Autodesk Inventor part; units mm, degrees
ref_plane "YZ Plane" through (0, 0, 0) normal (1, 0, 0) x (0, 1, 0)
ref_plane "XZ Plane" through (0, 0, 0) normal (0, 1, 0) x (-1, 0, 0)
ref_plane "XY Plane" through (0, 0, 0) normal (0, 0, 1) x (1, 0, 0)
sketch "Skizze1" plane through (0, 0, 0) normal (0, 0, 1) x (1, 0, 0)
  circle A0 centre (0, 0) radius 7.6
  line L0 (-22.5, 20) -> (-22.5, -20)
  line L1 (-22.5, -20) -> (-17.5, -20)
  line L2 (-17.5, -20) -> (-17.5, -10)
  line L3 (-22.5, 20) -> (-17.5, 20)
  line L4 (-17.5, 20) -> (-17.5, 10)
  line L5 (-17.5, 10) -> (0, 10)
  line L6 (-17.5, -10) -> (0, -10)
  arc A1 (0, -10) -> (0, 10) centre (0, 0) ccw
  dimension "d0" = 15.2
  dimension "d23" = 5
  dimension "d24" = 10
  dimension "d25" = 5
  dimension "d26" = 10
  dimension "d27" = 40
  dimension "d28" = 20
  dimension "d38" = 22.5
extrude "Extrusion1" add sketch "Skizze1" along normal blind 24
sketch "Skizze2" plane through (-22.5, -20, 0) normal (-1, 0, 0) x (0, 0, 1)
  line L0 (0, 40) -> (0, 0)
  line L1 (0, 0) -> (24, 0)
  line L2 (0, 40) -> (5, 40)
  line L3 (5, 40) -> (5, 0)
  line L4 (5, 0) -> (0, 0)
  line L5 (0, 0) -> (0, 40)
  point P0 (0, 20)
  dimension "d12" = 5
extrude "Extrusion2" add sketch "Skizze2" along normal blind 20
sketch "Skizze3" plane through (-22.5, -20, 5) normal (0, 0, 1) x (1, 0, 0)
  circle A0 centre (-10, 30) radius 1.6
  line L0 (0, 40) -> (-20, 40)
  line L1 (-20, 0) -> (-20, 40)
  circle A1 centre (-10, 10) radius 1.6
  line L2 (0, 0) -> (-20, 0)
  point P0 (22.5, 20)
  dimension "d15" = 3.2
  dimension "d16" = 10
  dimension "d17" = 10
  dimension "d18" = 3.2
  dimension "d19" = 10
  dimension "d20" = 10
extrude "Extrusion3" cut sketch "Skizze3" against normal through all
fillet "Rundung1" radius 2 6 edges at (-17.5, -10, 12) (-17.5, 10, 12) (-17.5, 20, 12) (-17.5, -20, 12) (-42.5, -20, 2.5) (-42.5, 20, 2.5)
sketch "Skizze4" plane through (-17.5, -18, 0) normal (1, 0, 0) x (0, 0, -1)
  circle A0 centre (-15, 3) radius 1.6
  circle A1 centre (-15, 33) radius 1.6
  line L0 (0, 0) -> (0, 6)
  line L1 (-24, -2) -> (0, -2)
  line L2 (-5, 38) -> (-24, 38)
  point P0 (0, 18)
  dimension "d30" = 3.2
  dimension "d31" = 3.2
  dimension "d32" = 15
  dimension "d33" = 5
  dimension "d34" = 15
  dimension "d35" = 5
extrude "Extrusion4" cut sketch "Skizze4" against normal through all
sketch "Skizze5" plane through (0, 0, 24) normal (0, 0, 1) x (1, 0, 0)
  circle A0 centre (0, 0) radius 7.6
  circle A1 centre (0, 0) radius 10
extrude "Extrusion5" add sketch "Skizze5" along normal blind 21
properties part number "flange" material "ABS-Kunststoff"
Source: CAD feature listing. Evaluate the final solid. Frame: model axes, mm. A direction names the side the tool comes from. Round coordinates to 2 decimals unless told otherwise and drop trailing zeros. Order: outer loops, then holes, each group sorted by start corner. A loop starts at its lowest first (then second) coordinate and runs counter-clockwise, first axis right, second up. Notation, with made-up numbers: (2, 46) -> (60, 46) arc R14 ccw to (60, 57) -> close; hole circle Ø8 at (-24, 48.5). An arc over 180 degrees is marked (long way). Use CSV: the item, a comma, the result in double quotes.
(1) Access query for faces 5 (the face through (-22.5, 0, 14)), 6 (the face through (9.282, -3.722, 27.185)), 7 (the face through (-17.5, -15, 12)), 8 (the face through (-42.5, 0, 2)). Directions: +Z, -Z, +X, -X, +Y, -Y. A direction counts if a zero-diameter tool reaches every point of the face in a straight line with its end or side. Return the directions, or none.
Report:
face 5,"+Z, -X, +Y, -Y"
face 6,"+Z"
face 7,"+Z, -Z, +X, -Y"
face 8,"+Z, -Z, -X, +Y, -Y"
(2) Section C-C on z = 4. Return the cut outline in (x, y), and give its area (3 significant figures).
Report:
outline,"(-42.5, -18) arc R2 ccw to (-40.5, -20) -> (-19.5, -20) arc R2 ccw to (-17.5, -18) -> (-17.5, -12) arc R2 cw to (-15.5, -10) -> (0, -10) arc R10 ccw to (0, 10) -> (-15.5, 10) arc R2 cw to (-17.5, 12) -> (-17.5, 18) arc R2 ccw to (-19.5, 20) -> (-40.5, 20) arc R2 ccw to (-42.5, 18) -> close; hole circle Ø3.2 at (-32.5, -10); hole circle Ø3.2 at (-32.5, 10); hole circle Ø15.2 at (0, 0)"
area,"1,310 mm^2"
(3) Section A-A on y = 0. Return the cut outline in (x, z), and give its area (3 significant figures).
Report:
outline,"(-42.5, 0) -> (-7.6, 0) -> (-7.6, 45) -> (-10, 45) -> (-10, 24) -> (-22.5, 24) -> (-22.5, 5) -> (-42.5, 5) -> close; (7.6, 0) -> (10, 0) -> (10, 45) -> (7.6, 45) -> close"
area,"616 mm^2"
(4) Section D-D on z = 21. Return the cut outline in (x, y), and give its area (3 significant figures).
Report:
outline,"(-22.5, -20) -> (-19.5, -20) arc R2 ccw to (-17.5, -18) -> (-17.5, -12) arc R2 cw to (-15.5, -10) -> (0, -10) arc R10 ccw to (0, 10) -> (-15.5, 10) arc R2 cw to (-17.5, 12) -> (-17.5, 18) arc R2 ccw to (-19.5, 20) -> (-22.5, 20) -> close; hole circle Ø15.2 at (0, 0)"
area,"526 mm^2"
(5) Section B-B on z = 15. Return the cut outline in (x, y).
Report:
outline,"(-22.5, -20) -> (-19.5, -20) arc R2 ccw to (-17.5, -18) -> (-17.5, -16.6) -> (-22.5, -16.6) -> close; (-22.5, -13.4) -> (-17.5, -13.4) -> (-17.5, -12) arc R2 cw to (-15.5, -10) -> (0, -10) arc R10 ccw to (0, 10) -> (-15.5, 10) arc R2 cw to (-17.5, 12) -> (-17.5, 13.4) -> (-22.5, 13.4) -> close; (-22.5, 16.6) -> (-17.5, 16.6) -> (-17.5, 18) arc R2 ccw to (-19.5, 20) -> (-22.5, 20) -> close; hole circle Ø15.2 at (0, 0)"
(6) Ray query, L1, parallel to Y at x = -20.6, z = 15; L2, parallel to Y at x = 0, z = 11; L3, parallel to Z at x = -28, y = -4. Return the intervals inside material, ascending.
Report:
L1,"-20 to -16.6, -13.4 to 13.4, 16.6 to 20"
L2,"-10 to -7.6, 7.6 to 10"
L3,"0 to 5"
(7) First-contact query: pin 1 Ø3 at (y, z) = (-10, 22) entering from -X; pin 2 Ø8 at (y, z) = (-6.5, 12) entering from +X; pin 3 Ø5 at (y, z) = (16, 7.5) entering from +X; pin 4 Ø2.5 at (x, y) = (-32.5, -10) entering from -Z. Flat tips, straight axial feed; report the tip coordinate or a pass-through.
Report:
pin 1,"x = -22.5"
pin 2,"x = 9.68"
pin 3,"x = -17.5"
pin 4,"through"
(8) Pull-direction query (Y, two-part tool) for faces 1 (the face through (-34.1, 10.07, 2.54)), 2 (the face through (-27.7, -20, 4.8)), 3 (the face through (-7.593, -0.334, 22.185)), 4 (the face through (-16.93, 10.6, 12.17)); classes: +Y half, -Y half, draft (parallel to the pull), parting line (faces both ways), or undercut.
Report:
face 1,"undercut"
face 2,"-Y half"
face 3,"undercut"
face 4,"+Y half"
